Read the model definition and answer for the solid it produces. Units are mm, in the model's axes. Round coordinates to 2 decimals unless told otherwise and drop trailing zeros. Order: outer loops, then holes, each group sorted by start corner. A loop starts at its lowest first (then second) coordinate and runs counter-clockwise, first axis right, second up. Notation, with made-up numbers: (9, 84.5) - (18, 84.5) arc R8 cw to (18, 93.5) - close; hole circle Ø10 at (48, 41). An arc over 180 degrees is marked (long way). One line per question, with ' | ' between items. Start each with the question number.
1) The part is cut by section B-B, the plane z = 12.5. Give the vertices of the cut face in (x, y).
2) Straight lines are drawn through the part: line 1 (Z direction, x = 4, y = -35.5); line 2 (Y direction, x = 5.75, z = 0.5); line 3 (Y direction, x = 5, z = 22.5). For each, find the intervals that lie inside material, in ascending order. Write a range as from..to.
3) The part is cut by section C-C, the plane x = 3.25. Count the separate pieces of the cut face and the enclosed holes in it, plus the area to 3 significant figures.
4) Flat-ended cylindrical pins translate along their axes: pin 1 (1.9 mm diameter, centred on x = 4, z = 7.5, fed in from -Y); pin 2 (1.5 mm diameter, centred on x = 5.5, y = 8.5, fed in from +Z). Find the tip coordinate at first contact, or state that the pin passes through.
5) The part is cut by section D-D, the plane y = 26. Give the vertices of the cut face in (x, z).
6) The part is cut by section A-A, the plane y = -53. Give the vertices of the cut face in (x, z).
from build123d import *

# Parameters (mm, degrees)
F0_W     = 38.1
F0_H     = 6.35
F1_DEPTH = 6.35
F2_R     = 6.35


with BuildPart() as f1:
    # F0 (on Right) → F1 (new body)
    with BuildSketch(Plane.YZ):
        Polygon((-44.45, 38.1), (-107.95, 38.1), (-107.95, 31.75), (-101.6, 31.75), (-101.6, 6.35), (-107.95, 6.35), (-107.95, -6.35), (-101.6, -6.35), (-101.6, -31.75), (-107.95, -31.75), (-107.95, -38.1), (107.95, -38.1), (107.95, -31.75), (101.6, -31.75), (101.6, -6.35), (107.95, -6.35), (107.95, 6.35), (101.6, 6.35), (101.6, 31.75), (107.95, 31.75), (107.95, 38.1), (44.45, 38.1), (44.45, -12.7), (-44.45, -12.7), align=None)
        with Locations((-50.8, -28.575)):
            Rectangle(F0_W, F0_H, mode=Mode.SUBTRACT)
        with Locations((50.8, -28.575)):
            Rectangle(F0_W, F0_H, mode=Mode.SUBTRACT)
    extrude(amount=F1_DEPTH)

    # F2
    f2_edges = [f1.edges().sort_by_distance(p)[0] for p in [
        (3.175, -44.45, 38.1),
        (3.175, -44.45, -12.7),
        (3.175, 44.45, 38.1),
        (3.175, 44.45, -12.7),
    ]]
    fillet(f2_edges, radius=F2_R)


solid = f1.part
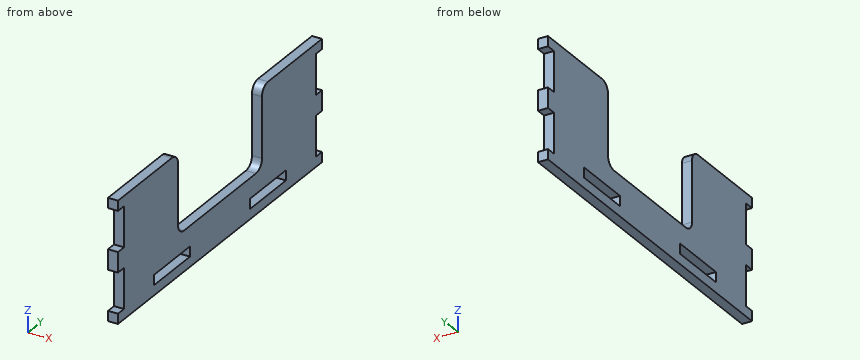
Values:
1) outline: (0, -101.6) - (6.35, -101.6) - (6.35, -44.45) - (0, -44.45) - close; (0, 44.45) - (6.35, 44.45) - (6.35, 101.6) - (0, 101.6) - close
2) line 1: z = -38.1..-31.75, -25.4..-12.7 | line 2: y = -107.95..-44.45, 44.45..107.95 | line 3: y = -101.6..-44.45, 44.45..101.6
3) separate pieces: 1 | enclosed holes: 2 | area: 10,800 mm^2
4) pin 1: stops at y = -101.6 | pin 2: stops at z = -12.7
5) outline: (0, -38.1) - (6.35, -38.1) - (6.35, -12.7) - (0, -12.7) - close
6) outline: (0, -38.1) - (6.35, -38.1) - (6.35, -31.75) - (0, -31.75) - close; (0, -25.4) - (6.35, -25.4) - (6.35, 38.1) - (0, 38.1) - close
